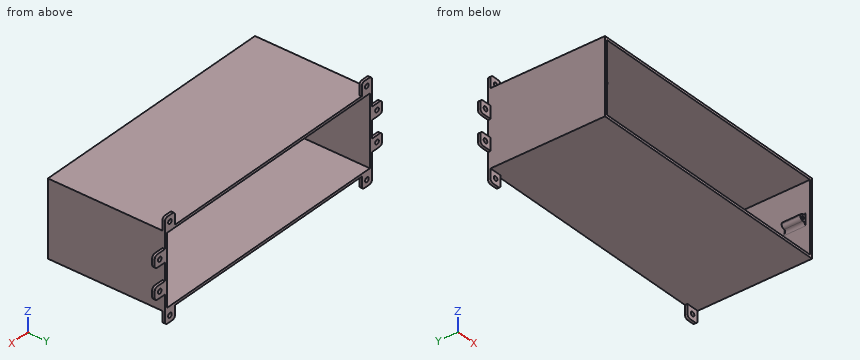
from build123d import *

# Parameters (mm, degrees)
F1_DEPTH     = 75
F0_W         = 8
F0_H         = 8
F0_R         = 1.425
F2_DEPTH     = 1.6
F3_R         = 2
F5_R         = 2
F6_START     = 60
F0_W_2       = 4
F0_H_2       = 4
F0_R_2       = 0.9
F6_DEPTH     = 12
F7_T1_DEPTH  = 12
F7_T6_DEPTH  = 4
F7_S7_R      = 0.9
F7_T8_DEPTH  = 4
F7_T13_DEPTH = 9
F7_T17_DEPTH = 17
F7_T24_DEPTH = 9
F7_T28_DEPTH = 17
F7_T31_DEPTH = 22
F9_R         = 2


# Not quite as in the source:
# - a fillet or chamfer that OpenCascade refuses, or shapes differently, is made with other operations: its cross-section is extruded or revolved along the edge and cut away or added


with BuildPart() as f1:
    # F0 (on Front) → F1 (new body)
    with BuildSketch(Plane.XZ):
        Polygon((-81.6, -13.6015841149), (-81.6, -24.1), (-73.6, -24.1), (73.6, -24.1), (81.6, -24.1), (81.6, -13.6015841149), (81.6, -5.6015841149), (81.6, 5.6015841149), (81.6, 13.6015841149), (81.6, 24.1), (73.6, 24.1), (-73.6, 24.1), (-81.6, 24.1), (-81.6, 13.6015841149), (-81.6, 5.6015841149), (-81.6, -5.6015841149), align=None)
        Polygon((80, -2), (80, -22.5), (-80, -22.5), (-80, 22.5), (80, 22.5), (80, 2), align=None, mode=Mode.SUBTRACT)
    extrude(amount=F1_DEPTH)

    # F0 (on Front) → F2 (join)
    with BuildSketch(Plane.XZ):
        Polygon((-81.6, -13.6015841149), (-81.6, -24.1), (-73.6, -24.1), (73.6, -24.1), (81.6, -24.1), (81.6, -13.6015841149), (81.6, -5.6015841149), (81.6, 5.6015841149), (81.6, 13.6015841149), (81.6, 24.1), (73.6, 24.1), (-73.6, 24.1), (-81.6, 24.1), (-81.6, 13.6015841149), (-81.6, 5.6015841149), (-81.6, -5.6015841149), align=None)
        Polygon((80, -2), (80, -22.5), (-80, -22.5), (-80, 22.5), (80, 22.5), (80, 2), align=None, mode=Mode.SUBTRACT)
        with Locations((-77.6, -28.1)):
            Rectangle(F0_W, F0_H)
        with Locations((-77.6, -28.1)):
            Circle(F0_R, mode=Mode.SUBTRACT)
        with Locations((-85.6, -9.6015841149)):
            Rectangle(F0_W, F0_H)
        with Locations((-85.6, -9.6015841149)):
            Circle(F0_R, mode=Mode.SUBTRACT)
        with Locations((77.6, -28.1)):
            Rectangle(F0_W, F0_H)
        with Locations((77.6, -28.1)):
            Circle(F0_R, mode=Mode.SUBTRACT)
        with Locations((-85.6, 9.6015841149)):
            Rectangle(F0_W, F0_H)
        with Locations((-85.6, 9.6015841149)):
            Circle(F0_R, mode=Mode.SUBTRACT)
        with Locations((85.6, -9.6015841149)):
            Rectangle(F0_W, F0_H)
        with Locations((85.6, -9.6015841149)):
            Circle(F0_R, mode=Mode.SUBTRACT)
        with Locations((-77.6, 28.1)):
            Rectangle(F0_W, F0_H)
        with Locations((-77.6, 28.1)):
            Circle(F0_R, mode=Mode.SUBTRACT)
        with Locations((85.6, 9.6015841149)):
            Rectangle(F0_W, F0_H)
        with Locations((85.6, 9.6015841149)):
            Circle(F0_R, mode=Mode.SUBTRACT)
        with Locations((77.6, 28.1)):
            Rectangle(F0_W, F0_H)
        with Locations((77.6, 28.1)):
            Circle(F0_R, mode=Mode.SUBTRACT)
    extrude(amount=F2_DEPTH)

    # F3
    f3_edges = [f1.edges().sort_by_distance(p)[0] for p in [
        (-81.6, -0.8, 32.1),
        (-73.6, -0.8, 32.1),
        (73.6, -0.8, 32.1),
        (81.6, -0.8, 32.1),
        (89.6, -0.8, -5.601584),
        (89.6, -0.8, -13.601584),
        (81.6, -0.8, -32.1),
        (73.6, -0.8, -32.1),
        (-89.6, -0.8, -13.601584),
        (-89.6, -0.8, -5.601584),
        (-81.6, -0.8, -32.1),
    ]]
    fillet(f3_edges, radius=F3_R)

    # F4: F1 across plane


with BuildPart() as f1_1:
    add(f1.part)
    add(f1.part.mirror(Plane.YZ))

    # F5
    f5_edges = [f1_1.edges().sort_by_distance(p)[0] for p in [
        (-73.6, -0.8, -32.1),
        (73.6, -0.8, -32.1),
    ]]
    fillet(f5_edges, radius=F5_R)

    # F0 (on Front) → F6 (join)
    with BuildSketch(Plane.XZ.offset(F6_START)):
        with Locations((78, 0)):
            Rectangle(F0_W_2, F0_H_2)
        with Locations((78, 0)):
            Circle(F0_R_2, mode=Mode.SUBTRACT)
    extrude(amount=F6_DEPTH)

    # F7: fillet of radius 2 on 5 edges, made by hand

    # F7_s2 → F7_t1 (join)
    with BuildSketch(Plane.XZ.offset(60)):
        with BuildLine():
            ThreePointArc((80, -4), (79.4142135624, -2.5857864376), (78, -2))
            Line((78, -2), (80, -2))
            Line((80, -2), (80, -4))
        make_face()
        with BuildLine():
            ThreePointArc((80, 4), (79.4142135624, 2.5857864376), (78, 2))
            Line((78, 2), (80, 2))
            Line((80, 2), (80, 4))
        make_face()
    extrude(amount=F7_T1_DEPTH)


with BuildPart() as f7_tool4:
    # F7_s5 → F7_t6 (new body)
    with BuildSketch(Plane.XY.offset(-2)):
        with BuildLine():
            ThreePointArc((80, -58), (79.4142135624, -59.4142135624), (78, -60))
            Line((78, -60), (80, -60))
            Line((80, -60), (80, -58))
        make_face()
    extrude(amount=F7_T6_DEPTH)

    # F7_s7 → F7_t8 (cut, symmetric)
    with BuildSketch(Plane.XZ.offset(59)):
        with Locations((78, 0)):
            Circle(F7_S7_R)
    extrude(amount=F7_T8_DEPTH, both=True, mode=Mode.SUBTRACT)


with BuildPart() as f1_2:
    add(f1_1.part)

    # F7_t3: union F7_tool4
    add(f7_tool4.part)


with BuildPart() as f7_tool11:
    # F7_s12 → F7_t13 (new body)
    with BuildSketch(Plane.XY.offset(-7)):
        with BuildLine():
            ThreePointArc((80, -58), (79.4142135624, -59.4142135624), (78, -60))
            Line((78, -60), (80, -60))
            Line((80, -60), (80, -58))
        make_face()
    extrude(amount=F7_T13_DEPTH)

    split(bisect_by=Plane.XY.offset(-2), keep=Keep.BOTTOM)


with BuildPart() as f7_tool15:
    # F7_s16 → F7_t17 (new body)
    with BuildSketch(Plane.XZ.offset(55)):
        with BuildLine():
            ThreePointArc((80, -4), (79.4142135624, -2.5857864376), (78, -2))
            Line((78, -2), (80, -2))
            Line((80, -2), (80, -4))
        make_face()
    extrude(amount=F7_T17_DEPTH)

    split(bisect_by=Plane.XZ.offset(60), keep=Keep.BOTTOM)


with BuildPart() as f7_tool11_1:
    add(f7_tool11.part)

    # F7_t19: intersect F7_tool15
    add(f7_tool15.part, mode=Mode.INTERSECT)


with BuildPart() as f1_3:
    add(f1_2.part)

    # F7_t9: union F7_tool11
    add(f7_tool11_1.part)


with BuildPart() as f7_tool22:
    # F7_s23 → F7_t24 (new body)
    with BuildSketch(Plane.XY.offset(-2)):
        with BuildLine():
            ThreePointArc((80, -58), (79.4142135624, -59.4142135624), (78, -60))
            Line((78, -60), (80, -60))
            Line((80, -60), (80, -58))
        make_face()
    extrude(amount=F7_T24_DEPTH)

    split(bisect_by=Plane.XY.offset(2), keep=Keep.TOP)


with BuildPart() as f7_tool26:
    # F7_s27 → F7_t28 (new body)
    with BuildSketch(Plane.XZ.offset(55)):
        with BuildLine():
            ThreePointArc((80, 4), (79.4142135624, 2.5857864376), (78, 2))
            Line((78, 2), (80, 2))
            Line((80, 2), (80, 4))
        make_face()
    extrude(amount=F7_T28_DEPTH)

    split(bisect_by=Plane.XZ.offset(60), keep=Keep.BOTTOM)


with BuildPart() as f7_tool22_1:
    add(f7_tool22.part)

    # F7_t30: intersect F7_tool26
    add(f7_tool26.part, mode=Mode.INTERSECT)


with BuildPart() as f1_4:
    add(f1_3.part)

    # F7_t20: union F7_tool22
    add(f7_tool22_1.part)

    # F7_s32 → F7_t31 (cut)
    with BuildSketch(Plane.XZ.offset(55)):
        with BuildLine():
            ThreePointArc((78, -2), (76.5857864376, -1.4142135624), (76, 0))
            Line((76, 0), (76, -2))
            Line((76, -2), (78, -2))
        make_face()
        with BuildLine():
            ThreePointArc((78, 2), (76.5857864376, 1.4142135624), (76, 0))
            Line((76, 0), (76, 2))
            Line((76, 2), (78, 2))
        make_face()
    extrude(amount=F7_T31_DEPTH, mode=Mode.SUBTRACT)

    # F8: F1 across plane


with BuildPart() as f1_5:
    add(f1_4.part)
    add(f1_4.part.mirror(Plane.YZ))

    # F9
    f9_edges = [f1_5.edges().sort_by_distance(p)[0] for p in [
        (89.6, -0.8, 5.601584),
        (89.6, -0.8, 13.601584),
        (-89.6, -0.8, 5.601584),
        (-89.6, -0.8, 13.601584),
    ]]
    fillet(f9_edges, radius=F9_R)


solid = f1_5.part
Input: part model. Units: mm. Frame: model coordinates. Coordinates: 2 decimals unless noted, no trailing zeros. Order: outer loops, then holes, each group sorted by start corner. A loop starts at its lowest first (then second) coordinate and runs counter-clockwise, first axis right, second up. Notation, with made-up numbers: M -8,83 L 39,83 A6 cw 39,88 Z; hole C 47.5,48.25 d9. An arc over 180 degrees is marked long. Write item = value, one per line. Start each with the question number.
(1) Line query: line 1 along X through (y, z) = (-1, 28); line 2 along Z through (x, y) = (-85.6, -0.6); line 3 along Z through (x, y) = (78, -67). Output: solid intervals per line, ascending. Write a range as [from, to].
(2) First-contact query: P1, Ø1, axis at x = -35, y = -20, coming from the +Z side; P2, Ø4, axis at x = -86.5, z = -10, coming from the -Y side; P3, Ø1.7, axis at x = 77.6, z = 28.1, coming from the +Y side; P4, Ø12, axis at y = -22, z = -2.5, coming from the +X side. Flat tips, straight axial feed; report the tip coordinate or a pass-through.
(3) Section A-A on x = 0. Output: boundary loops of the cut face in (y, z), and give its area (3 significant figures).
(4) Section B-B on y = -25.5. Output: boundary loops of the cut face in (x, z), and give its area (3 significant figures).
Result set:
q1.line_1 = [-81.6, -79.02], [-76.18, -73.6], [73.6, 76.18], [79.02, 81.6]
q1.line_2 = [-13.6, -11.03], [-8.18, -5.6], [5.6, 8.18], [11.03, 13.6]
q1.line_3 = [-24.1, -22.5], [-2, -0.9], [0.9, 2], [22.5, 24.1]
q2.P1 = 24.1
q2.P2 = -1.6
q2.P3 = through
q2.P4 = 81.6
q3.outline = M -75,-24.1 L 0,-24.1 L 0,-22.5 L -75,-22.5 Z; M -75,22.5 L 0,22.5 L 0,24.1 L -75,24.1 Z
q3.area = 240 mm²
q4.outline = M -81.6,-24.1 L 81.6,-24.1 L 81.6,24.1 L -81.6,24.1 Z; hole M -80,-22.5 L 80,-22.5 L 80,22.5 L -80,22.5 Z
q4.area = 666 mm²
